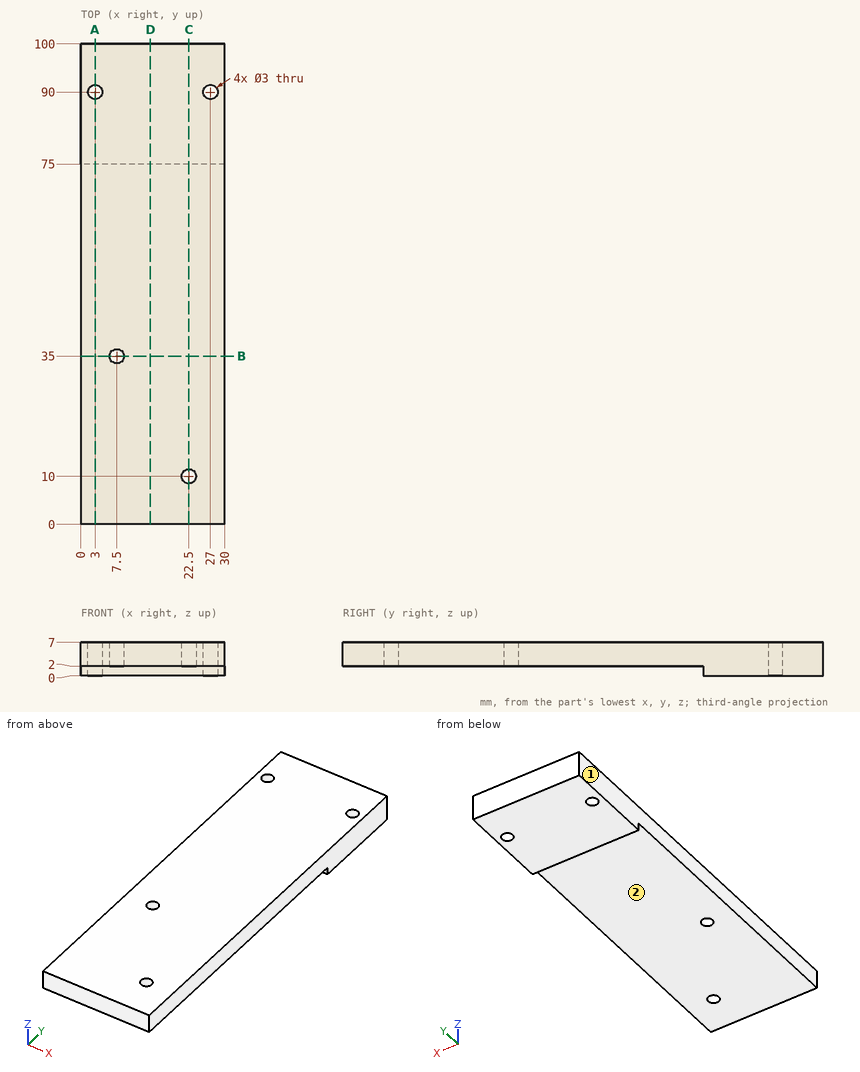
Geometry: see drawing. Coordinates: mm, zero at the bounding-box minimum. A direction names the side the tool comes from. Round coordinates to 2 decimals unless told otherwise and drop trailing zeros. Loops run counter-clockwise (first coordinate to the right, second up) from the corner with the lowest first, then second, coordinate; pieces in that order, holes last. Notation, with made-up numbers: (-0.5, 66.5) - (49.5, 66.5) arc R25 cw to (49.5, 92.5) - close; hole circle Ø6 at (-31.5, 16.25). An arc over 180 degrees is marked (long way). Write item = value, one per line. Start each with the question number.
(1) Pin query (flat end, axial travel): pin 1 (3 mm diameter, centred on x = 16.5, y = 26.5, fed in from -Z). Return the tip coordinate at first contact, or that it passes through.
(2) Ray query, line 1 along X through (y, z) = (90, 2.75); line 2 along X through (y, z) = (10, 5.25); line 3 along Y through (x, z) = (3, 4.5). Return the intervals inside material, ascending. Write a range as from..to.
(3) Section query D-D, the plane x = 14.5. Output: boundary loops of the cut face in (y, z).
(4) Section query C-C, the plane x = 22.5. Output: boundary loops of the cut face in (y, z).
(5) Set-up query: the marked faces 1 and 2. Return all of +Z, -Z, +X, -X, +Y, -Y with unobstructed straight access to the full face (end or side cutting, diameter ignored); none if empty.
(6) Section query B-B, the plane y = 35. Output: boundary loops of the cut face in (x, z).
(7) Section query A-A, the plane x = 3. Output: boundary loops of the cut face in (y, z).
Conclusion:
q1.pin_1 = 2
q2.line_1 = 0..1.5, 4.5..25.5, 28.5..30
q2.line_2 = 0..21, 24..30
q2.line_3 = 0..88.5, 91.5..100
q3.outline = (0, 2) - (75, 2) - (75, 0) - (100, 0) - (100, 7) - (0, 7) - close
q4.outline = (0, 2) - (8.5, 2) - (8.5, 7) - (0, 7) - close; (11.5, 2) - (75, 2) - (75, 0) - (100, 0) - (100, 7) - (11.5, 7) - close
q5.face_1 = +Z, -Z, -X, +Y, -Y
q5.face_2 = -Z, +X, -X, -Y
q6.outline = (0, 2) - (6, 2) - (6, 7) - (0, 7) - close; (9, 2) - (30, 2) - (30, 7) - (9, 7) - close
q7.outline = (0, 2) - (75, 2) - (75, 0) - (88.5, 0) - (88.5, 7) - (0, 7) - close; (91.5, 0) - (100, 0) - (100, 7) - (91.5, 7) - close
